Geometry check sheet. Reference: the model listing, model coordinates, mm. A direction names the side the tool comes from. Round coordinates to 2 decimals unless told otherwise and drop trailing zeros. Order: outer loops, then holes, each group sorted by start corner. A loop starts at its lowest first (then second) coordinate and runs counter-clockwise, first axis right, second up. Notation, with made-up numbers: (85, 76) - (104, 76) arc R11 ccw to (104, 88) - close; hole circle Ø7 at (18.5, -22.75). An arc over 180 degrees is marked (long way). Return JSON: item names as keys, results as strings. Group by question number.
Q1. Gauge pin test, flat end, axial feed: pin 1 Ø1 at (x, y) = (200, -179.5) entering from +Z. Record the tip position at first contact, or that the pin passes through.
Q2. Sectioned sample at B-B, the plane z = 17. Record the cut outline in (x, y) (3 decimals).
Q3. Draft check along Z on faces 4 (the flat face through (225, -226, 63.5)), 5 (the flat face through (63, -136.525, 31)), 6 (the flat face through (225, -122, -25.4)), 7 (the flat face through (249, -226, 53.975)). Enter one of: pulls with the +Z half, pulls with the -Z half, needs draft (parallel to the pull), parting line crosses it, or undercut.
Q4. Tool access check on faces 1 (the flat face through (226, -31.75, 32)), 2 (the flat face through (247, -226, 41.275)), 3 (the flat face through (225, 0, 20)). Record the directions out of +Z, -Z, +X, -X, +Y, -Y that give a thin tool (end or side, any length) a straight path to the whole face; none if there is none.
Q5. Sectioned sample at A-A, the plane x = 221.5. Record the cut outline in (y, z) (3 decimals), then the cut area to 3 significant figures.
Q6. Material ranges on line 1 along Y through (x, z) = (68.5, 60.5) (3 decimals); line 2 along Z through (x, y) = (63.5, -227.5); line 3 along Y through (x, z) = (281, 58), recorded low to high.
Q7. Sectioned sample at D-D, the plane y = -215.5. Record the cut outline in (x, z) (3 decimals).
Q8. Sectioned sample at C-C, the plane x = 407.5. Record the cut outline in (y, z), then the cut area to 3 significant figures.
```python
from build123d import *

# Parameters (mm, degrees)
F0_W      = 457.2
F0_H      = 63.5
F1_DEPTH  = 31.75
F2_W      = 31.75
F2_H      = 63.5
F3_DEPTH  = 177.8
F4_W      = 31.75
F4_H      = 63.5
F4_W_2    = 425.45
F5_DEPTH  = 31.75
F6_W      = 31.75
F6_H      = 63.5
F7_DEPTH  = 177.8
F8_W      = 15.875
F8_H      = 63.5
F9_DEPTH  = 63.5
F10_R     = 3.175
F11_DEPTH = 190.5
F12_W     = 457.2
F12_H     = 241.3
F13_DEPTH = 25.4
F15_DEPTH = 254
F16_R     = 5.08


with BuildPart() as f1:
    # F0 (on Front) → F1 (new body)
    with BuildSketch(Plane.XZ):
        with Locations((228.6, 31.75)):
            Rectangle(F0_W, F0_H)
    extrude(amount=F1_DEPTH)

    # F2 (on face) → F3 (join)
    with BuildSketch(Plane.XZ.offset(31.75)):
        with Locations((441.325, 31.75)):
            Rectangle(F2_W, F2_H)
    extrude(amount=F3_DEPTH)

    # F4 (on face) → F5 (join)
    with BuildSketch(Plane.XZ.offset(209.55)):
        with Locations((441.325, 31.75)):
            Rectangle(F4_W, F4_H)
        with Locations((212.725, 31.75)):
            Rectangle(F4_W_2, F4_H)
    extrude(amount=F5_DEPTH)

    # F6 (on face) → F7 (join)
    with BuildSketch(Plane.XZ.offset(31.75)):
        with Locations((15.875, 31.75)):
            Rectangle(F6_W, F6_H)
    extrude(amount=F7_DEPTH)

    # F8 (on face) → F9 (join)
    with BuildSketch(Plane.YZ.offset(31.75)):
        with Locations((-128.5875, 31.75)):
            Rectangle(F8_W, F8_H)
        with Locations((-112.7125, 31.75)):
            Rectangle(F8_W, F8_H)
    extrude(amount=F9_DEPTH)

    # F10 (on face) → F11 (cut, symmetric)
    with BuildSketch(Plane.XZ.offset(136.525)):
        with Locations((63.5, 47.625)):
            Circle(F10_R)
    extrude(amount=F11_DEPTH, both=True, mode=Mode.SUBTRACT)

    # F12 (on face) → F13 (join)
    with BuildSketch(Plane(origin=(0, 0, 0), x_dir=(1, 0, 0), z_dir=(0, 0, -1))):
        with Locations((228.6, 120.65)):
            Rectangle(F12_W, F12_H)
        Polygon((425.45, 209.55), (425.45, 31.75), (31.75, 31.75), (31.75, 104.775), (95.25, 104.775), (95.25, 136.525), (31.75, 136.525), (31.75, 209.55), align=None, mode=Mode.SUBTRACT)
        Polygon((31.75, 31.75), (425.45, 31.75), (425.45, 209.55), (31.75, 209.55), (31.75, 136.525), (95.25, 136.525), (95.25, 104.775), (31.75, 104.775), align=None)
    extrude(amount=F13_DEPTH)

    # F14 (on face) → F15 (cut)
    with BuildSketch(Plane.XZ.offset(241.3)):
        Polygon((314.325, 53.975), (247.65, 53.975), (180.975, 53.975), (180.975, 41.275), (314.325, 41.275), align=None)
    extrude(amount=-F15_DEPTH, mode=Mode.SUBTRACT)

    # F16
    f16_edges = [f1.edges().sort_by_distance(p)[0] for p in [
        (180.975, -225.425, 41.275),
        (180.975, -225.425, 53.975),
        (314.325, -225.425, 41.275),
        (314.325, -225.425, 53.975),
        (180.975, -15.875, 41.275),
        (180.975, -15.875, 53.975),
        (314.325, -15.875, 41.275),
        (314.325, -15.875, 53.975),
    ]]
    fillet(f16_edges, radius=F16_R)


solid = f1.part
```
Reply:
{
 "1": {"pin 1": "z = 0"},
 "2": {"outline": "(0, -241.3) - (457.2, -241.3) - (457.2, 0) - (0, 0) - close; hole (31.75, -209.55) - (425.45, -209.55) - (425.45, -31.75) - (31.75, -31.75) - (31.75, -104.775) - (95.25, -104.775) - (95.25, -136.525) - (31.75, -136.525) - close"},
 "3": {"face 4": "pulls with the +Z half", "face 5": "needs draft", "face 6": "pulls with the -Z half", "face 7": "undercut"},
 "4": {"face 1": "+Z", "face 2": "+Y, -Y", "face 3": "+Z, -Z, +X, -X, +Y"},
 "5": {"outline": "(-241.3, -25.4) - (0, -25.4) - (0, 41.275) - (-31.75, 41.275) - (-31.75, 0) - (-209.55, 0) - (-209.55, 41.275) - (-241.3, 41.275) - close; (-241.3, 53.975) - (-209.55, 53.975) - (-209.55, 63.5) - (-241.3, 63.5) - close; (-31.75, 53.975) - (0, 53.975) - (0, 63.5) - (-31.75, 63.5) - close", "area": "9,350 mm^2"},
 "6": {"line 1": "-241.3 to -209.55, -136.525 to -104.775, -31.75 to 0", "line 2": "-25.4 to 44.45, 50.8 to 63.5", "line 3": "-241.3 to -209.55, -31.75 to 0"},
 "7": {"outline": "(0, -25.4) - (457.2, -25.4) - (457.2, 63.5) - (0, 63.5) - close; hole circle Ø6.35 at (63.5, 47.625); hole (180.975, 46.355) arc R5.08 ccw to (186.055, 41.275) - (309.245, 41.275) arc R5.08 ccw to (314.325, 46.355) - (314.325, 48.895) arc R5.08 ccw to (309.245, 53.975) - (186.055, 53.975) arc R5.08 ccw to (180.975, 48.895) - close"},
 "8": {"outline": "(-241.3, -25.4) - (0, -25.4) - (0, 63.5) - (-31.75, 63.5) - (-31.75, 0) - (-209.55, 0) - (-209.55, 63.5) - (-241.3, 63.5) - close", "area": "10,200 mm^2"}
}
